```python
from build123d import *

# Parameters (mm, degrees)
SKETCH_W     = 38.1
SKETCH_H     = 38.1
SKETCH_R     = 1.125
PAD_DEPTH    = 1.6
PAD001_DEPTH = 7.3
SKETCH002_R  = 7.5
PAD002_DEPTH = 14.5
SKETCH003_W  = 10
SKETCH003_H  = 4.5
PAD003_DEPTH = 6.25


with BuildPart() as part:
    # Sketch → Pad (new body)
    with BuildSketch(Plane.XY):
        Rectangle(SKETCH_W, SKETCH_H)
        with Locations((-14, 14)):
            Circle(SKETCH_R, mode=Mode.SUBTRACT)
        with Locations((14, 14)):
            Circle(SKETCH_R, mode=Mode.SUBTRACT)
        with Locations((14, -14)):
            Circle(SKETCH_R, mode=Mode.SUBTRACT)
        with Locations((-14, -14)):
            Circle(SKETCH_R, mode=Mode.SUBTRACT)
        with Locations((-17, 17)):
            Circle(SKETCH_R, mode=Mode.SUBTRACT)
        with Locations((17, 17)):
            Circle(SKETCH_R, mode=Mode.SUBTRACT)
        with Locations((17, -17)):
            Circle(SKETCH_R, mode=Mode.SUBTRACT)
        with Locations((-17, -17)):
            Circle(SKETCH_R, mode=Mode.SUBTRACT)
    extrude(amount=-PAD_DEPTH)

    # Sketch001 → Pad001 (join)
    with BuildSketch(Plane.XY):
        with BuildLine():
            Line((-8, 2.25), (-8, 8))
            Line((-8, 8), (8, 8))
            Line((8, 8), (8, 2.25))
            Line((8, 2.25), (10.000011, 2.25))
            ThreePointArc((10.000011, -2.25), (12.25, 0), (10.000011, 2.25))
            Line((8, -2.25), (10.000011, -2.25))
            Line((8, -8), (8, -2.25))
            Line((-8, -8), (8, -8))
            Line((-8, -2.25), (-8, -8))
            Line((-9.999989, -2.25), (-8, -2.25))
            ThreePointArc((-10, 2.25), (-12.25, -6e-06), (-9.999989, -2.25))
            Line((-10, 2.25), (-8, 2.25))
        make_face()
    extrude(amount=PAD001_DEPTH)

    # Sketch002 (on DatumPlane) → Pad002 (join)
    with BuildSketch(Plane.XY.offset(7.3)):
        Circle(SKETCH002_R)
    extrude(amount=PAD002_DEPTH)

    # Sketch003 (on DatumPlane) → Pad003 (join)
    with BuildSketch(Plane(origin=(0, 0, -1.6), x_dir=(1, 0, 0), z_dir=(0, 0, -1))):
        with Locations((5, 13.25)):
            Rectangle(SKETCH003_W, SKETCH003_H)
    extrude(amount=PAD003_DEPTH)


solid = part.part
```
Input: part model. Units: mm. Frame: model coordinates. A direction names the side the tool comes from. Coordinates: 2 decimals unless noted, no trailing zeros. Order: outer loops, then holes, each group sorted by start corner. A loop starts at its lowest first (then second) coordinate and runs counter-clockwise, first axis right, second up. Notation, with made-up numbers: (-15.75, -20.75) - (28.25, -20.75) arc R15 cw to (28.25, -3.75) - close; hole circle Ø7 at (82, 23). An arc over 180 degrees is marked (long way). Put each result on its own line as item: value.
1. Reachability of faces 1 (the face through (5, -15.5, -5)), 2 (the face through (-7.493, 0.33, 14.448)), 3 (the face through (10, -13, -5)) from +Z, -Z, +X, -X, +Y, -Y: full face, straight path, thin tool, end or side. Return the list, or none.
Report:
face 1: -Z, +X, -X, -Y
face 2: +Z
face 3: -Z, +X, +Y, -Y
2. Contact query for flat-ended pins moving along their axis: pin 1 Ø1.5 at (x, y) = (-10, -1.5) entering from +Z; pin 2 Ø0.6 at (x, z) = (9.5, 3.5) entering from -Y; pin 3 Ø1 at (y, z) = (-0.5, 13.5) entering from +X; pin 4 Ø5 at (x, z) = (-11, 18) entering from -Y. Output: stop coordinate, or through.
Report:
pin 1: stops at z = 7.3
pin 2: stops at y = -2.25
pin 3: stops at x = 7.5
pin 4: passes through
3. Cut plane B-B on y = -14. Return the cut outline in (x, z) (3 decimals), then the cut area to 3 significant figures.
Report:
outline: (-19.05, -1.6) - (-15.125, -1.6) - (-15.125, 0) - (-19.05, 0) - close; (-12.875, -1.6) - (0, -1.6) - (0, -7.85) - (10, -7.85) - (10, -1.6) - (12.875, -1.6) - (12.875, 0) - (-12.875, 0) - close; (15.125, -1.6) - (19.05, -1.6) - (19.05, 0) - (15.125, 0) - close
area: 116 mm2
4. Draft query along X for faces 4 (the face through (-16.4, 17.95, -0.79)), 5 (the face through (6, 5, 7.3)), 6 (the face through (17.6, 17.95, -0.79)), 7 (the face through (-8, -5, 4)). Return one class per face: pulls with the +X half, pulls with the -X half, needs draft (parallel to the pull), parting line crosses it, or undercut.
Report:
face 4: undercut
face 5: needs draft
face 6: undercut
face 7: pulls with the -X half
5. Cut plane C-C on z = 5.5. Return the cut outline in (x, y).
Report:
outline: (-10, -2.25) - (-8, -2.25) - (-8, -8) - (8, -8) - (8, -2.25) - (10, -2.25) arc R2.25 ccw to (10, 2.25) - (8, 2.25) - (8, 8) - (-8, 8) - (-8, 2.25) - (-10, 2.25) arc R2.25 ccw to start
6. Cut plane D-D on y = 3. Return the cut outline in (x, z), then the cut area to 3 significant figures.
Report:
outline: (-19.05, -1.6) - (19.05, -1.6) - (19.05, 0) - (8, 0) - (8, 7.3) - (6.87, 7.3) - (6.87, 21.8) - (-6.87, 21.8) - (-6.87, 7.3) - (-8, 7.3) - (-8, 0) - (-19.05, 0) - close
area: 377 mm2
7. Line query: line 1 along Y through (x, z) = (-17, -1) (3 decimals); line 2 along Y through (x, z) = (14, -1.25) (3 decimals); line 3 along Z through (x, y) = (-10.5, -7). Output: solid intervals per line, ascending.
Report:
line 1: y = -19.05 to -18.125, -15.875 to 15.875, 18.125 to 19.05
line 2: y = -19.05 to -15.125, -12.875 to 12.875, 15.125 to 19.05
line 3: z = -1.6 to 0
8. Cut plane A-A on x = -14. Return the cut outline in (y, z) (3 decimals).
Report:
outline: (-19.05, -1.6) - (-15.125, -1.6) - (-15.125, 0) - (-19.05, 0) - close; (-12.875, -1.6) - (12.875, -1.6) - (12.875, 0) - (-12.875, 0) - close; (15.125, -1.6) - (19.05, -1.6) - (19.05, 0) - (15.125, 0) - close
